Geometry: see drawing. Coordinates: mm, zero at the bounding-box minimum. Round coordinates to 2 decimals unless told otherwise and drop trailing zeros. Loops run counter-clockwise (first coordinate to the right, second up) from the corner with the lowest first, then second, coordinate; pieces in that order, holes last. Notation, with made-up numbers: M 44.25,2.5 L 52.25,2.5 A23 cw 52.25,29.5 Z; hole C 60.25,14.5 d3. An arc over 180 degrees is marked long. Answer as a JSON object with one key per item and string values.
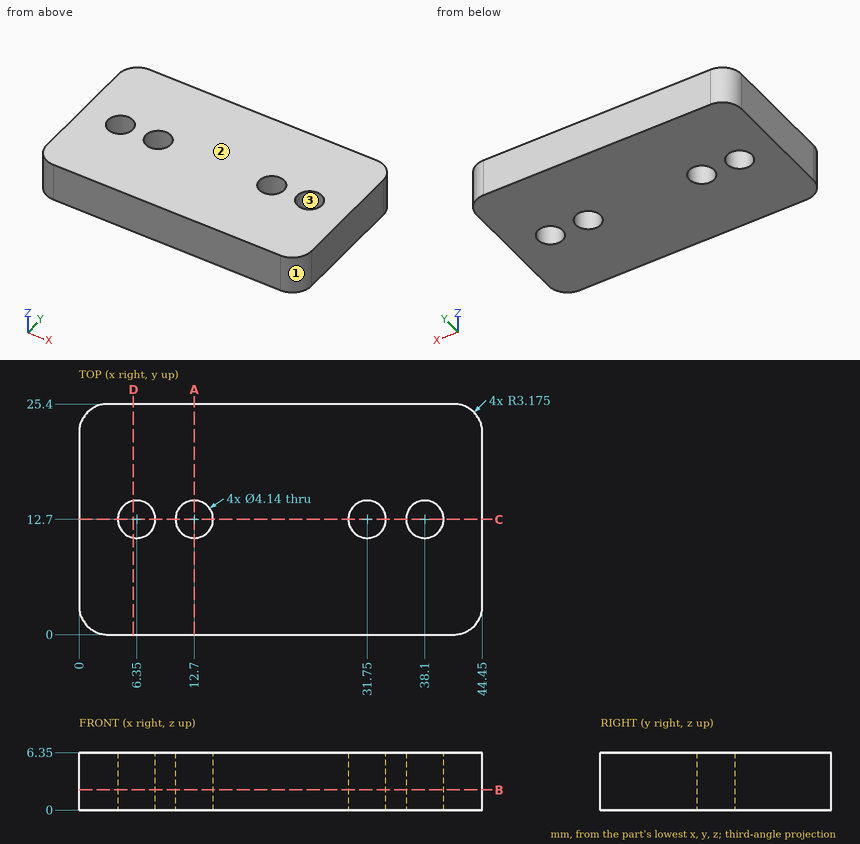
1) Section query C-C (y = 12.7). Return the cut outline in (x, z).
Results:
{"outline": "M 0,0 L 4.28,0 L 4.28,6.35 L 0,6.35 Z; M 8.42,0 L 10.63,0 L 10.63,6.35 L 8.42,6.35 Z; M 14.77,0 L 29.68,0 L 29.68,6.35 L 14.77,6.35 Z; M 33.82,0 L 36.03,0 L 36.03,6.35 L 33.82,6.35 Z; M 40.17,0 L 44.45,0 L 44.45,6.35 L 40.17,6.35 Z"}
2) Section query D-D (x = 6). Return the cut outline in (y, z), and give its area (3 significant figures).
Results:
{"outline": "M 0,0 L 10.66,0 L 10.66,6.35 L 0,6.35 Z; M 14.74,0 L 25.4,0 L 25.4,6.35 L 14.74,6.35 Z", "area": "135 mm2"}
3) Ray query, line 1 (Y direction, x = 31.75, z = 2.25); line 2 (X direction, y = 11.5, z = 4); line 3 (Y direction, x = 36.5, z = 0.75). Return the intervals inside material, ascending.
Results:
{"line 1": "0 to 10.63, 14.77 to 25.4", "line 2": "0 to 4.66, 8.04 to 11.01, 14.39 to 30.06, 33.44 to 36.41, 39.79 to 44.45", "line 3": "0 to 11.39, 14.01 to 25.4"}
4) Section query A-A (x = 12.7). Return the cut outline in (y, z), and give its area (3 significant figures).
Results:
{"outline": "M 0,0 L 10.63,0 L 10.63,6.35 L 0,6.35 Z; M 14.77,0 L 25.4,0 L 25.4,6.35 L 14.77,6.35 Z", "area": "135 mm2"}
5) Pin query (flat end, axial travel): P1, Ø3.5, axis at x = 12.7, y = 12.7, coming from the +Z side. Return the tip coordinate at first contact, or that it passes through.
Results:
{"P1": "through"}
6) Pull-direction query (Y, two-part tool) for the marked faces 1, 2 and 3; classes: +Y half, -Y half, draft (parallel to the pull), parting line (faces both ways), or undercut.
Results:
{"face 1": "-Y half", "face 2": "draft", "face 3": "undercut"}
7) Section query B-B (z = 2.25). Count the separate pieces of the cut face and the enclosed holes in it, and give its area (3 significant figures).
Results:
{"separate pieces": "1", "enclosed holes": "4", "area": "1,070 mm2"}
